from build123d import *

# Parameters (mm, degrees)
SKETCH1_R           = 11
SKETCH1_R_2         = 2
BOSS_EXTRUDE1_DEPTH = 10
BOSS_EXTRUDE2_START = -3
SKETCH2_R           = 11
SKETCH2_R_2         = 7.5
BOSS_EXTRUDE2_DEPTH = 3


with BuildPart() as part:
    # Sketch1 → Boss-Extrude1 (new body)
    with BuildSketch(Plane(origin=(0, 0, 0), x_dir=(1, 0, 0), z_dir=(0, 1, 0))):
        with BuildLine():
            Line((-2.5, 17.031832941), (-13.5, 10.68097998))
            ThreePointArc((-13.5, 10.68097998), (-15.330127019, 8.850852961), (-16, 6.350852961))
            Line((-16, 6.350852961), (-16, -6.350852961))
            ThreePointArc((-16, -6.350852961), (-15.330127019, -8.850852961), (-13.5, -10.68097998))
            Line((-13.5, -10.68097998), (-2.5, -17.031832941))
            ThreePointArc((-2.5, -17.031832941), (0, -17.701705922), (2.5, -17.031832941))
            Line((2.5, -17.031832941), (13.5, -10.68097998))
            ThreePointArc((13.5, -10.68097998), (15.330127019, -8.850852961), (16, -6.350852961))
            Line((16, -6.350852961), (16, 6.350852961))
            ThreePointArc((16, 6.350852961), (15.330127019, 8.850852961), (13.5, 10.68097998))
            Line((13.5, 10.68097998), (2.5, 17.031832941))
            ThreePointArc((2.5, 17.031832941), (0, 17.701705922), (-2.5, 17.031832941))
        make_face()
        with Locations(Location((0, 0, 0), (0, 0, 270))):
            Circle(SKETCH1_R, mode=Mode.SUBTRACT)
        with Locations(Location((0, 13.5, 0), (0, 0, 270))):
            Circle(SKETCH1_R_2, mode=Mode.SUBTRACT)
        with Locations(Location((11.691342951, 6.75, 0), (0, 0, 270))):
            Circle(SKETCH1_R_2, mode=Mode.SUBTRACT)
        with Locations(Location((11.691342951, -6.75, 0), (0, 0, 270))):
            Circle(SKETCH1_R_2, mode=Mode.SUBTRACT)
        with Locations(Location((0, -13.5, 0), (0, 0, 270))):
            Circle(SKETCH1_R_2, mode=Mode.SUBTRACT)
        with Locations(Location((-11.691342951, -6.75, 0), (0, 0, 270))):
            Circle(SKETCH1_R_2, mode=Mode.SUBTRACT)
        with Locations(Location((-11.691342951, 6.75, 0), (0, 0, 270))):
            Circle(SKETCH1_R_2, mode=Mode.SUBTRACT)
    extrude(amount=BOSS_EXTRUDE1_DEPTH)

    # Sketch2 → Boss-Extrude2 (add)
    with BuildSketch(Plane(origin=(0, 10, 0), x_dir=(1, 0, 0), z_dir=(0, 1, 0)).offset(BOSS_EXTRUDE2_START)):
        with Locations(Location((0, 0, 0), (0, 0, 270))):
            Circle(SKETCH2_R)
        with Locations(Location((0, 0, 0), (0, 0, 270))):
            Circle(SKETCH2_R_2, mode=Mode.SUBTRACT)
    extrude(amount=BOSS_EXTRUDE2_DEPTH)


solid = part.part
Can you work these out from the model? Positions are in its coordinate system, mm. A direction names the side the tool comes from. Give positions to 0.01 mm unless a question says otherwise; leave off trailing zeros. Loops run counter-clockwise (first coordinate to the right, second up) from the corner with the lowest first, then second, coordinate; pieces in that order, holes last. Notation, with made-up numbers: (33, -21) - (75, -21) arc R18 cw to (75, 5) - close; hole circle Ø1 at (63, 53.25). An arc over 180 degrees is marked (long way). Return JSON: item names as keys, results as strings.
1. I want a section at B-B on z = 0. Please give me the cut outline in (x, y).
Output values:
{"outline": "(-16, 0) - (-11, 0) - (-11, 7) - (-7.5, 7) - (-7.5, 10) - (-16, 10) - close; (7.5, 7) - (11, 7) - (11, 0) - (16, 0) - (16, 10) - (7.5, 10) - close"}
2. I want a section at D-D on x = -6.5. Please give me the cut outline in (y, z), and give its area (3 significant figures).
Output values:
{"outline": "(0, -14.72) - (10, -14.72) - (10, -3.74) - (7, -3.74) - (7, -8.87) - (0, -8.87) - close; (0, 8.87) - (7, 8.87) - (7, 3.74) - (10, 3.74) - (10, 14.72) - (0, 14.72) - close", "area": "148 mm²"}
3. We'd pull the mould along X, two halves only. Please class faces 3 (the face through (0, 10, -8)), 4 (the face through (-10.74, 3.45, -2.38)), 5 (the face through (0.33, 8.479, -7.493)), 6 (the face through (8.1, 4.9, -13.8)): +X half, -X half, draft (parallel to the pull), parting line (faces both ways), or undercut.
Output values:
{"face 3": "draft", "face 4": "undercut", "face 5": "undercut", "face 6": "+X half"}
4. For faces 1 (the face through (2.6, 7, 7.2)), 2 (the face through (13.674, 4.93, 6.49)), which set-ups out of +Z, -Z, +X, -X, +Y, -Y let a thin tool reach every point of the face, with its end or its side?
Output values:
{"face 1": "-Y", "face 2": "+Y, -Y"}
5. I want a section at C-C on z = -6.75. Please give me the cut outline in (x, y).
Output values:
{"outline": "(-15.98, 0) - (-13.69, 0) - (-13.69, 10) - (-15.98, 10) - close; (-9.69, 0) - (-8.69, 0) - (-8.69, 7) - (-3.27, 7) - (-3.27, 10) - (-9.69, 10) - close; (3.27, 7) - (8.69, 7) - (8.69, 0) - (9.69, 0) - (9.69, 10) - (3.27, 10) - close; (13.69, 0) - (15.98, 0) - (15.98, 10) - (13.69, 10) - close"}
6. I want a section at A-A on x = 0. Please give me the cut outline in (y, z).
Output values:
{"outline": "(0, -17.7) - (10, -17.7) - (10, -15.5) - (0, -15.5) - close; (0, -11.5) - (10, -11.5) - (10, -7.5) - (7, -7.5) - (7, -11) - (0, -11) - close; (0, 11) - (7, 11) - (7, 7.5) - (10, 7.5) - (10, 11.5) - (0, 11.5) - close; (0, 15.5) - (10, 15.5) - (10, 17.7) - (0, 17.7) - close"}
7. I'm going to push flat-ended pins straight in: pin 1 Ø1.5 at (x, y) = (6, 3) entering from +Z; pin 2 Ø5 at (x, z) = (-4, -4.5) entering from +Y; pin 3 Ø3.5 at (x, z) = (11.69, -6.75) entering from +Y; pin 4 Ø6 at (x, z) = (-5, -5.5) entering from -Y. Where does each tip first touch, or does it pass through?
Output values:
{"pin 1": "stops at z = 15.44", "pin 2": "stops at y = 10", "pin 3": "passes through", "pin 4": "stops at y = 7"}
8. If I drill on line 1 (Z direction, x = -1, y = 1.25); line 2 (X direction, y = 8.55, z = 0); line 3 (X direction, y = 6.25, z = 0), over which ranges is the centre line in solid material (lowest first)?
Output values:
{"line 1": "z = -17.6 to -15.23, -11.77 to -10.95, 10.95 to 11.77, 15.23 to 17.6", "line 2": "x = -16 to -7.5, 7.5 to 16", "line 3": "x = -16 to -11, 11 to 16"}
